Work out the finished part from the listing and answer in its coordinate system (mm). Face numbers are marked on the shaded views. A direction names the side the tool comes from. Give positions to 0.01 mm unless a question says otherwise; leave off trailing zeros. Order: outer loops, then holes, each group sorted by start corner. A loop starts at its lowest first (then second) coordinate and runs counter-clockwise, first axis right, second up.
```python
from build123d import *

# Parameters (mm, degrees)
F2_R     = 3.05
F3_DEPTH = 13
F4_R     = 0.5
F5_R     = 1.2
F6_DEPTH = 7
F7_R     = 1.5
F8_DEPTH = 13


with BuildPart() as f1:
    # F0 (on Front) → F1 (revolve)
    with BuildSketch(Plane.XZ):
        Polygon((-5, 0), (0, 0), (0, 15), (-6.5, 15), (-6.5, 0), align=None)
    revolve(axis=Axis((0, 0, -3.667768), (0, 0, -1)))

    # F2 (on face) → F3 (cut)
    with BuildSketch(Plane(origin=(0, 0, 0), x_dir=(1, 0, 0), z_dir=(0, 0, -1))):
        Circle(F2_R)
    extrude(amount=-F3_DEPTH, mode=Mode.SUBTRACT)

    # F4
    f4_edges = [f1.edges().sort_by_distance(p)[0] for p in [
        (6.5, 0, 15),
    ]]
    fillet(f4_edges, radius=F4_R)

    # F5 (on Front) → F6 (cut)
    with BuildSketch(Plane.XZ):
        with Locations((0, 9)):
            Circle(F5_R)
    extrude(amount=F6_DEPTH, mode=Mode.SUBTRACT)

    # F7 (on face) → F8 (cut)
    with BuildSketch(Plane(origin=(0, 0, 0), x_dir=(1, 0, 0), z_dir=(0, 0, -1))):
        with Locations((-7.5, 0)):
            Circle(F7_R)
        with Locations((-6.495191, -3.75)):
            Circle(F7_R)
        with Locations((-3.75, -6.495191)):
            Circle(F7_R)
        with Locations((0, -7.5)):
            Circle(F7_R)
        with Locations((3.75, -6.495191)):
            Circle(F7_R)
        with Locations((6.495191, -3.75)):
            Circle(F7_R)
        with Locations((7.5, 0)):
            Circle(F7_R)
        with Locations((6.495191, 3.75)):
            Circle(F7_R)
        with Locations((3.75, 6.495191)):
            Circle(F7_R)
        with Locations((0, 7.5)):
            Circle(F7_R)
        with Locations((-3.75, 6.495191)):
            Circle(F7_R)
        with Locations((-6.495191, 3.75)):
            Circle(F7_R)
    extrude(amount=-F8_DEPTH, mode=Mode.SUBTRACT)


solid = f1.part
```
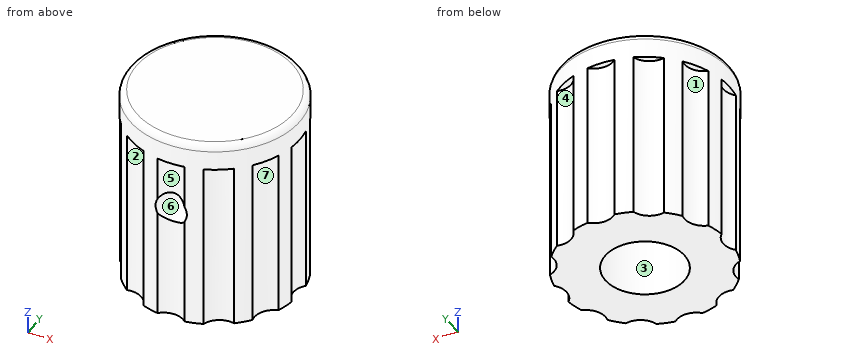
1. The part is cut by section A-A (x = 0). Write down the section's boundary in (y, z), then the cut area to 3 significant figures.
Findings below:
outline: (-6.5, 13) - (-6, 13) - (-6, 10.2) - (-3.05, 10.2) - (-3.05, 13) - (3.05, 13) - (3.05, 0) - (6, 0) - (6, 13) - (6.5, 13) - (6.5, 14.5) arc R0.5 ccw to (6, 15) - (-6, 15) arc R0.5 ccw to (-6.5, 14.5) - close; (-6, 0) - (-3.05, 0) - (-3.05, 7.8) - (-6, 7.8) - close
area: 95.5 mm2
2. The mould has two halves that part along Y. Classify the marked faces 5, 6 and 7: pulls with the +Y half, pulls with the -Y half, needs draft (parallel to the pull), parting line crosses it, or undercut.
Findings below:
face 5: pulls with the -Y half
face 6: needs draft
face 7: undercut
3. The part is cut by section D-D (z = 9). Write down the section's boundary in (x, y), then the cut area to 3 significant figures.
Findings below:
outline: (-6.42, -1.04) arc R6.5 ccw to (-6.08, -2.31) arc R1.5 cw to (-5.04, -4.11) arc R6.5 ccw to (-4.11, -5.04) arc R1.5 cw to (-2.31, -6.08) arc R6.5 ccw to (-1.2, -6.39) - (-1.2, -2.8) arc R3.05 cw (long way) to (1.2, -2.8) - (1.2, -6.39) arc R6.5 ccw to (2.31, -6.08) arc R1.5 cw to (4.11, -5.04) arc R6.5 ccw to (5.04, -4.11) arc R1.5 cw to (6.08, -2.31) arc R6.5 ccw to (6.42, -1.04) arc R1.5 cw to (6.42, 1.04) arc R6.5 ccw to (6.08, 2.31) arc R1.5 cw to (5.04, 4.11) arc R6.5 ccw to (4.11, 5.04) arc R1.5 cw to (2.31, 6.08) arc R6.5 ccw to (1.04, 6.42) arc R1.5 cw to (-1.04, 6.42) arc R6.5 ccw to (-2.31, 6.08) arc R1.5 cw to (-4.11, 5.04) arc R6.5 ccw to (-5.04, 4.11) arc R1.5 cw to (-6.08, 2.31) arc R6.5 ccw to (-6.42, 1.04) arc R1.5 cw to start
area: 87.3 mm2
4. The part is cut by section B-B (y = 0). Write down the section's boundary in (x, z).
Findings below:
outline: (-6.5, 13) - (-6, 13) - (-6, 0) - (-3.05, 0) - (-3.05, 13) - (3.05, 13) - (3.05, 0) - (6, 0) - (6, 13) - (6.5, 13) - (6.5, 14.5) arc R0.5 ccw to (6, 15) - (-6, 15) arc R0.5 ccw to (-6.5, 14.5) - close
5. Given P1, Ø5, axis at x = -1, z = 8, coming from the +Y side; P2, Ø6, axis at y = 4.5, z = 10, coming from the -X side; P3, Ø1.5, axis at y = 4, z = 8.5, coming from the -X side, each flat-ended and moving along its own axis, determine where each tip first touches the part or whether it passes through.
Findings below:
P1: stops at y = 6.42
P2: stops at x = -6.32
P3: stops at x = -5.08
6. Straight lines are drawn through the part: probe 1 along X at (y, z) = (-3.8, 9); probe 2 along X at (y, z) = (0, 3). For each, find the intervals that lie inside material, in ascending order.
Findings below:
probe 1: x = -5 to -1.2, 1.2 to 5
probe 2: x = -6 to -3.05, 3.05 to 6
7. Which of the six approach directions +Z, -Z, +X, -X, +Y, -Y give full straight-line access (tool end or side, diameter ignored) to the marked faces 1, 2, 3 and 4?
Findings below:
face 1: -Z, -X
face 2: -Z, -Y
face 3: -Z
face 4: -Z, +Y
8. The part is cut by section C-C (z = 2.75). Write down the section's boundary in (x, y), then the cut area to 3 significant figures.
Findings below:
outline: (-6.42, -1.04) arc R6.5 ccw to (-6.08, -2.31) arc R1.5 cw to (-5.04, -4.11) arc R6.5 ccw to (-4.11, -5.04) arc R1.5 cw to (-2.31, -6.08) arc R6.5 ccw to (-1.04, -6.42) arc R1.5 cw to (1.04, -6.42) arc R6.5 ccw to (2.31, -6.08) arc R1.5 cw to (4.11, -5.04) arc R6.5 ccw to (5.04, -4.11) arc R1.5 cw to (6.08, -2.31) arc R6.5 ccw to (6.42, -1.04) arc R1.5 cw to (6.42, 1.04) arc R6.5 ccw to (6.08, 2.31) arc R1.5 cw to (5.04, 4.11) arc R6.5 ccw to (4.11, 5.04) arc R1.5 cw to (2.31, 6.08) arc R6.5 ccw to (1.04, 6.42) arc R1.5 cw to (-1.04, 6.42) arc R6.5 ccw to (-2.31, 6.08) arc R1.5 cw to (-4.11, 5.04) arc R6.5 ccw to (-5.04, 4.11) arc R1.5 cw to (-6.08, 2.31) arc R6.5 ccw to (-6.42, 1.04) arc R1.5 cw to start; hole circle Ø6.1 at (0, 0)
area: 95.0 mm2
